```python
from build123d import *

# Parameters (mm, degrees)
F0_W      = 12.6
F0_H      = 23
F1_DEPTH  = 22.5
F3_W      = 12.6
F3_H      = 32.4
F4_DEPTH  = 2.4
F5_R      = 1.05
F6_DEPTH  = 25
F7_R      = 6.3
F8_DEPTH  = 4.2
F9_R      = 2.3
F10_DEPTH = 6.7


with BuildPart() as f1:
    # F0 (on Front) → F1 (new body)
    with BuildSketch(Plane.XZ):
        with Locations((0, 5.2)):
            Rectangle(F0_W, F0_H)
    extrude(amount=F1_DEPTH)

    # F3 (on offset) → F4 (join)
    with BuildSketch(Plane.XZ.offset(6.7)):
        with Locations((0, 5.2)):
            Rectangle(F3_W, F3_H)
    extrude(amount=-F4_DEPTH)

    # F5 (on offset) → F6 (cut)
    with BuildSketch(Plane.XZ.offset(6.7)):
        with Locations((0, 19.1)):
            Circle(F5_R)
        with Locations((0, -8.7)):
            Circle(F5_R)
    extrude(amount=-F6_DEPTH, mode=Mode.SUBTRACT)

    # F7 (on Front) → F8 (join)
    with BuildSketch(Plane.XZ):
        Circle(F7_R)
    extrude(amount=-F8_DEPTH)

    # F9 (on Front) → F10 (join)
    with BuildSketch(Plane.XZ):
        Circle(F9_R)
    extrude(amount=-F10_DEPTH)


solid = f1.part
```
Geometry check sheet. Reference: the model listing, model coordinates, mm. A direction names the side the tool comes from. Give positions to 0.01 mm unless a question says otherwise; leave off trailing zeros. Order: outer loops, then holes, each group sorted by start corner. A loop starts at its lowest first (then second) coordinate and runs counter-clockwise, first axis right, second up. Notation, with made-up numbers: (32.5, 57.5) -> (77.5, 57.5) arc R14 ccw to (77.5, 72.5) -> close; hole circle Ø10 at (49.5, 77). An arc over 180 degrees is marked (long way). Write each question's results on one line, items separated by ' | '. Start each with the question number.
(1) Access from +Z, -Z, +X, -X, +Y, -Y to the whole of each face (thin tool, end or side, straight path). Record for faces 5 (the face through (5, 0, -5)), 6 (the face through (-1.825, 5.432, -1.4)), 7 (the face through (0, -2, -6.3)).
(2) Sectioned sample at B-B (x = -1.5). Enter the section's corners in (y, z).
(3) Sectioned sample at C-C (z = 5). Enter the section's corners in (x, y).
(4) Sectioned sample at A-A (z = 19.1). Enter the section's corners in (x, y), plus the area to 3 significant figures.
(5) Gauge pin test, flat ends, axial feed: P1, Ø5, axis at x = -3, y = -10, coming from the +Z side; P2, Ø5, axis at x = -4.5, z = -4.5, coming from the +Y side; P3, Ø6, axis at x = -2.5, y = -17.5, coming from the -Z side; P4, Ø4, axis at x = -1.5, z = -7.5, coming from the -Y side. Record the tip position at first contact, or that the pin passes through.
(6) Sectioned sample at D-D (y = -10.5). Enter the section's corners in (x, z), plus the area to 3 significant figures.
(7) Mould release check, pull along X, two halves, no side actions. Record for faces 1 (the face through (-0.228, -5.517, 18.075)), 2 (the face through (0, -14, -6.3)), 3 (the face through (-5, 2.07, -3.83)), 4 (the face through (-6.3, -11, 5)): pulls with the +X half, pulls with the -X half, needs draft (parallel to the pull), parting line crosses it, or undercut.
(8) Scan lines: line 1 (Z direction, x = 0, y = -5.4); line 2 (X direction, y = -4.75, z = 19); line 3 (Y direction, x = 4.5, z = 11). Record each from-to range of solid material in increasing order.
Answer below:
1) face 5: -Z, +X, +Y | face 6: +Y | face 7: -Z, +X, -X, +Y
2) outline: (-22.5, -6.3) -> (-6.7, -6.3) -> (-6.7, -11) -> (-4.3, -11) -> (-4.3, -6.3) -> (0, -6.3) -> (0, -6.12) -> (4.2, -6.12) -> (4.2, -1.74) -> (6.7, -1.74) -> (6.7, 1.74) -> (4.2, 1.74) -> (4.2, 6.12) -> (0, 6.12) -> (0, 16.7) -> (-4.3, 16.7) -> (-4.3, 21.4) -> (-6.7, 21.4) -> (-6.7, 16.7) -> (-22.5, 16.7) -> close
3) outline: (-6.3, -22.5) -> (6.3, -22.5) -> (6.3, 0) -> (3.83, 0) -> (3.83, 4.2) -> (-3.83, 4.2) -> (-3.83, 0) -> (-6.3, 0) -> close
4) outline: (-6.3, -6.7) -> (-1.05, -6.7) -> (-1.05, -4.3) -> (-6.3, -4.3) -> close; (1.05, -6.7) -> (6.3, -6.7) -> (6.3, -4.3) -> (1.05, -4.3) -> close | area: 25.2 mm2
5) P1: z = 16.7 | P2: y = 4.2 | P3: z = -6.3 | P4: y = -22.5
6) outline: (-6.3, -6.3) -> (6.3, -6.3) -> (6.3, 16.7) -> (-6.3, 16.7) -> close | area: 290 mm2
7) face 1: undercut | face 2: needs draft | face 3: parting line crosses it | face 4: pulls with the -X half
8) line 1: -11 to -9.75, -7.65 to 18.05, 20.15 to 21.4 | line 2: -6.3 to -1.05, 1.05 to 6.3 | line 3: -22.5 to 0
